from build123d import *

# Parameters (mm, degrees)
F0_R     = 7.5
F0_R_2   = 5
F1_DEPTH = 2
F0_R_3   = 3
F2_DEPTH = 33


# Not quite as in the source:
# - a fillet or chamfer that OpenCascade refuses, or shapes differently, is made with other operations: its cross-section is extruded or revolved along the edge and cut away or added


with BuildPart() as f1:
    # F0 (on Top) → F1 (new body)
    with BuildSketch(Plane.XY):
        Circle(F0_R)
        Circle(F0_R_2, mode=Mode.SUBTRACT)
    extrude(amount=F1_DEPTH)

    # F0 (on Top) → F2 (join)
    with BuildSketch(Plane.XY):
        Circle(F0_R_2)
        Circle(F0_R_3, mode=Mode.SUBTRACT)
    extrude(amount=F2_DEPTH)

    # F3: fillet of radius 3 on 2 edges, made by hand

    # F3_s1 → F3_t2 (revolve, cut)
    with BuildSketch(Plane.XZ):
        with BuildLine():
            ThreePointArc((6, 0), (3.8786796564, 0.8786796564), (3, 3))
            Line((3, 3), (3, 0))
            Line((3, 0), (6, 0))
        make_face()
    revolve(axis=Axis((0, 0, 0), (0, 0, 1)), mode=Mode.SUBTRACT)

    # F3_s3 → F3_t4 (revolve, cut)
    with BuildSketch(Plane.XZ):
        with BuildLine():
            ThreePointArc((3, 30.1715728753), (3.5505102572, 31.9036236828), (5, 33))
            Line((5, 33), (3, 33))
            Line((3, 33), (3, 30.1715728753))
        make_face()
    revolve(axis=Axis((0, 0, 33), (0, 0, 1)), mode=Mode.SUBTRACT)


solid = f1.part
Geometry check sheet. Reference: the model listing, model coordinates, mm. A direction names the side the tool comes from. Give positions to 0.01 mm unless a question says otherwise; leave off trailing zeros. Loops run counter-clockwise (first coordinate to the right, second up) from the corner with the lowest first, then second, coordinate; pieces in that order, holes last. Notation, with made-up numbers: M 21,8.5 L 27,8.5 A19 ccw 27,31.5 Z; hole C 2.5,58.25 d8. An arc over 180 degrees is marked long. Answer as a JSON object with one key per item and string values. Group by question number.
Item 1: Access from +Z, -Z, +X, -X, +Y, -Y to the whole of each face (thin tool, end or side, straight path). Record for faces 4 (the flat face through (2, 6, 0)), 5 (the cylindrical face through (-1.08, -4.88, 17.28)).
Item 2: Gauge pin test, flat ends, axial feed: pin 1 (7.5 mm diameter, centred on x = 0.5, y = 1, fed in from +Z); pin 2 (8 mm diameter, centred on y = -3, z = 23.5, fed in from +X); pin 3 (5 mm diameter, centred on x = -2, z = 7.5, fed in from -Y). Record the tip position at first contact, or that the pin passes through.
Item 3: Material ranges on L1, parallel to Y at x = 0, z = 16.25; L2, parallel to X at y = 2.5, z = 26; L3, parallel to Z at x = 2.5, y = -7, recorded low to high.
Item 4: Sectioned sample at C-C on z = 24.5. Record the boundary of the cut face in (x, y).
Item 5: Mould release check, pull along X, two halves, no side actions. Record for faces 1 (the flat face through (2, -5, 2)), 2 (the cylindrical face through (-3, 0, 16)), 3 (the cylindrical face through (-7.493, 0.33, 0.986)): pulls with the +X half, pulls with the -X half, needs draft (parallel to the pull), parting line crosses it, or undercut.
Item 6: Sectioned sample at A-A on y = 0. Record the boundary of the cut face in (x, z).
Findings below:
{
 "1": {"face 4": "-Z, +X, -X, +Y, -Y", "face 5": "+Z"},
 "2": {"pin 1": "z = 32.95", "pin 2": "x = 5", "pin 3": "y = -5"},
 "3": {"L1": "-5 to -3, 3 to 5", "L2": "-4.33 to -1.66, 1.66 to 4.33", "L3": "0 to 2"},
 "4": {"outline": "C 0,0 d10; hole C 0,0 d6"},
 "5": {"face 1": "needs draft", "face 2": "undercut", "face 3": "parting line crosses it"},
 "6": {"outline": "M -7.5,0 L -6,0 A3 ccw -3,3 L -3,30.17 A3 ccw -5,33 L -5,2 L -7.5,2 Z; M 3,3 A3 ccw 6,0 L 7.5,0 L 7.5,2 L 5,2 L 5,33 A3 ccw 3,30.17 Z"}
}
